from build123d import *

# Parameters (mm, degrees)
SALIENTE_EXTRUIR2_DEPTH = 4


with BuildPart() as part:
    # Croquis1 → Saliente-Extruir2 (new body)
    with BuildSketch(Plane.XY):
        with BuildLine():
            Line((50, -100.385371697), (50, -94.385371697))
            ThreePointArc((50, -94.385371697), (59.472562128, -93.35362238), (68.500882915, -90.306761094))
            ThreePointArc((68.500882915, -90.306761094), (70.539255421, -86.910059757), (74.500570941, -86.932902716))
            ThreePointArc((74.500570941, -86.932902716), (93.999774318, -50.244446404), (74.265957135, -13.681648121))
            ThreePointArc((74.265957135, -13.681648121), (70.072325001, -13.890235332), (68.002756877, -10.23688798))
            ThreePointArc((68.002756877, -10.23688798), (59.205072417, -7.35902347), (50, -6.385371697))
            Line((50, -6.385371697), (50, -0.385371697))
            ThreePointArc((50, -0.385371697), (100, -50.385371697), (50, -100.385371697))
        make_face()
    extrude(amount=SALIENTE_EXTRUIR2_DEPTH)


solid = part.part
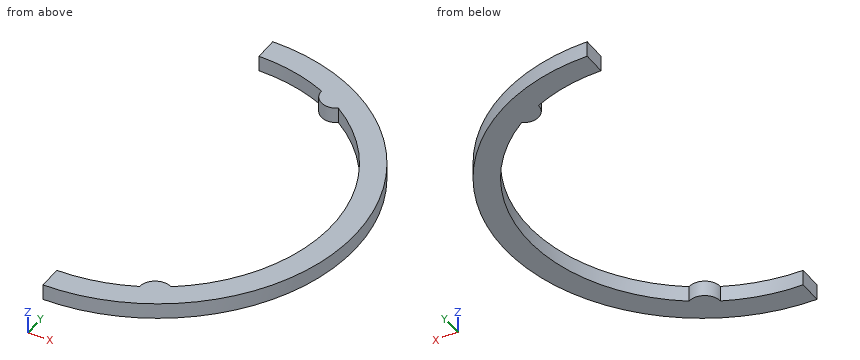
Part model, mm, in its own coordinate system. Give positions to 0.01 mm unless a question says otherwise; leave off trailing zeros. Loops run counter-clockwise (first coordinate to the right, second up) from the corner with the lowest first, then second, coordinate; pieces in that order, holes last.
(1) Band-saw the part on C-C (x = 60.5). Write the cut outline in (y, z), and give its area (3 significant figures).
Return value:
outline: (-99.27, 0) - (-93.11, 0) - (-93.11, 4) - (-99.27, 4) - close; (-7.66, 0) - (-1.5, 0) - (-1.5, 4) - (-7.66, 4) - close
area: 49.3 mm2
(2) Band-saw the part on A-A (x = 88). Write the cut outline in (y, z).
Return value:
outline: (-82.88, 0) - (-72.57, 0) - (-72.57, 4) - (-82.88, 4) - close; (-28.2, 0) - (-17.89, 0) - (-17.89, 4) - (-28.2, 4) - close
(3) Band-saw the part on B-B (z = 2.3). Write the cut outline in (x, y), and give its area (3 significant figures).
Return value:
outline: (50, -100.39) arc R50 ccw to (50, -0.39) - (50, -6.39) arc R44 cw to (68, -10.24) arc R4 ccw to (74.27, -13.68) arc R44 cw to (74.5, -86.93) arc R4 ccw to (68.5, -90.31) arc R44 cw to (50, -94.39) - close
area: 908 mm2
(4) Drill centre lines: line 1 along Y through (x, z) = (82.5, 2.2); line 2 along Y through (x, z) = (89, 3.15); line 3 along X through (y, z) = (-38, 0.35). Where is each one in solid material? Low to high.
Return value:
line 1: y = -88.38 to -80.05, -20.72 to -12.39
line 2: y = -81.67 to -70.76, -30.01 to -19.1
line 3: x = 92.22 to 98.44
(5) Pin check, flat tips, straight feed: pin 1 (12 mm diameter, centred on x = 83.5, y = -22.5, fed in from +Z); pin 2 (2 mm diameter, centred on y = -45.5, z = 0.5, fed in from -X); pin 3 (1 mm diameter, centred on x = 84, z = 1, fed in from -Y); pin 4 (1.5 mm diameter, centred on y = -39.5, z = 3, fed in from -X). Stop position of each tip, or through.
Return value:
pin 1: stops at z = 4
pin 2: stops at x = 93.6
pin 3: stops at y = -87.5
pin 4: stops at x = 92.43
(6) Band-saw the part on D-D (y = -75.5). Write the cut outline in (x, z), and give its area (3 significant figures).
Return value:
outline: (86.13, 0) - (93.23, 0) - (93.23, 4) - (86.13, 4) - close
area: 28.4 mm2
